```python
from build123d import *

# Parameters (mm, degrees)
F0_W      = 908.05
F0_H      = 34.925
F1_DEPTH  = 2032
F2_W      = 601.726
F2_H      = 615.442
F3_DEPTH  = 34.926
F8_DEPTH  = 926.592
F9_DEPTH  = 615.442
F11_DEPTH = 34.926
F13_DEPTH = 908.05
F15_DEPTH = 34.926
F17_W     = 506.7300000006
F17_H     = 34.925
F18_DEPTH = 831.596
F19_W     = 506.7300000008
F19_H     = 34.925
F20_DEPTH = 520.446


with BuildPart() as f1:
    # F0 (on Top) → F1 (new body)
    with BuildSketch(Plane.XY):
        with Locations((-454.025, 17.4625)):
            Rectangle(F0_W, F0_H)
    extrude(amount=F1_DEPTH)

    # F2 (on Front) → F3 (cut, through all)
    with BuildSketch(Plane.XZ):
        Polygon((-754.888, 1917.446), (-754.888, 990.854), (-153.162, 990.854), (-153.162, 1917.446), (-454.025, 1917.446), align=None)
        with Locations((-454.025, 510.921)):
            Rectangle(F2_W, F2_H)
    extrude(amount=-F3_DEPTH, mode=Mode.SUBTRACT)

    # F6 (on face) → F8 (join, through all)
    with BuildSketch(Plane(origin=(0, 0, 1917.446), x_dir=(1, 0, 0), z_dir=(0, 0, -1))):
        Polygon((-200.66, -17.4625), (-200.66, -34.925), (-186.8149014921, -24.003), (-176.911, -24.003), (-167.0070985079, -24.003), (-153.162, -34.925), (-153.162, -17.4625), (-153.162, 0), (-167.0070985079, -10.922), (-176.911, -10.922), (-186.8149014921, -10.922), (-200.66, 0), align=None)
        Polygon((-741.0429014921, -24.003), (-731.139, -24.003), (-721.2350985079, -24.003), (-707.39, -34.925), (-707.39, -17.4625), (-707.39, 0), (-721.2350985079, -10.922), (-731.139, -10.922), (-741.0429014921, -10.922), (-754.888, 0), (-754.888, -17.4625), (-754.888, -34.925), align=None)
    extrude(amount=F8_DEPTH)

    # F7 (on face) → F9 (join, through all)
    with BuildSketch(Plane.XY.offset(203.2)):
        Polygon((-200.66, 34.925), (-200.66, 17.4625), (-200.66, 0), (-186.8149014921, 10.922), (-176.911, 10.922), (-167.0070985079, 10.922), (-153.162, 0), (-153.162, 17.4625), (-153.162, 34.925), (-167.0070985079, 24.003), (-176.911, 24.003), (-186.8149014921, 24.003), align=None)
        Polygon((-721.2350985079, 24.003), (-731.139, 24.003), (-741.0429014921, 24.003), (-754.888, 34.925), (-754.888, 17.4625), (-754.888, 0), (-741.0429014921, 10.922), (-731.139, 10.922), (-721.2350985079, 10.922), (-707.39, 0), (-707.39, 17.4625), (-707.39, 34.925), align=None)
    extrude(amount=F9_DEPTH)

    # F10 (on Front) → F11 (cut, through all)
    with BuildSketch(Plane.XZ):
        Polygon((-754.888, 1917.446), (-454.025, 1616.583), (-153.162, 1917.446), (-200.66, 1917.446), (-707.39, 1917.446), align=None)
        Polygon((-153.162, 990.854), (-454.025, 1291.717), (-754.888, 990.854), (-200.66, 990.854), align=None)
        Polygon((-153.162, 818.642), (-200.66, 818.642), (-707.39, 818.642), (-754.888, 818.642), (-454.025, 517.779), align=None)
        Polygon((-754.888, 203.2), (-200.66, 203.2), (-153.162, 203.2), (-454.025, 504.063), align=None)
    extrude(amount=-F11_DEPTH, mode=Mode.SUBTRACT)


with BuildPart() as f13:
    # F12 (on Right) → F13 (new body, through all)
    with BuildSketch(Plane.YZ):
        Polygon((34.925, 1917.446), (0, 1917.446), (10.9219999999, 1903.6009014923), (10.922, 1883.7930985079), (0, 1869.948), (34.925, 1869.948), (24.003, 1883.793098508), (24.003, 1903.6009014921), align=None)
    extrude(amount=-F13_DEPTH)


with BuildPart() as f13b:
    # F12 (on Right) → F13, piece 2 (new body, through all)
    with BuildSketch(Plane.YZ):
        Polygon((10.922, 1004.6990985079), (0, 990.854), (34.925, 990.854), (24.0029999999, 1004.6990985081), (24.003, 1024.5069014921), (34.925, 1038.3520000001), (0, 1038.352), (10.922, 1024.5069014922), align=None)
    extrude(amount=-F13_DEPTH)


with BuildPart() as f13c:
    # F12 (on Right) → F13, piece 3 (new body, through all)
    with BuildSketch(Plane.YZ):
        Polygon((24.003, 784.9890985079), (24.003, 804.7969014922), (34.925, 818.642), (0, 818.642), (10.922, 804.796901492), (10.922, 784.9890985079), (1e-10, 771.1440000001), (34.925, 771.144), align=None)
    extrude(amount=-F13_DEPTH)


with BuildPart() as f13d:
    # F12 (on Right) → F13, piece 4 (new body, through all)
    with BuildSketch(Plane.YZ):
        Polygon((34.925, 203.2), (24.003, 217.0450985079), (24.003, 236.852901492), (34.925, 250.698), (0, 250.698), (10.922, 236.8529014921), (10.922, 217.0450985078), (0, 203.2), align=None)
    extrude(amount=-F13_DEPTH)


with BuildPart() as f15_tool:
    # F14 (on Front) → F15 (new body, through all)
    with BuildSketch(Plane.XZ):
        Polygon((-754.888, 818.642), (-754.888, 203.2), (-454.025, 504.063), (-153.162, 203.2), (-153.162, 818.642), (-454.025, 517.779), align=None)
        Polygon((-153.162, 1917.446), (-454.025, 1616.583), (-754.888, 1917.446), (-754.888, 990.854), (-454.025, 1291.717), (-153.162, 990.854), align=None)
    extrude(amount=-F15_DEPTH)


with BuildPart() as f13_1:
    add(f13.part)

    # F15: cut by f15_tool
    add(f15_tool.part, mode=Mode.SUBTRACT)


with BuildPart() as f13b_1:
    add(f13b.part)

    # F15: cut by f15_tool
    add(f15_tool.part, mode=Mode.SUBTRACT)


with BuildPart() as f13c_1:
    add(f13c.part)

    # F15: cut by f15_tool
    add(f15_tool.part, mode=Mode.SUBTRACT)


with BuildPart() as f13d_1:
    add(f13d.part)

    # F15: cut by f15_tool
    add(f15_tool.part, mode=Mode.SUBTRACT)


with BuildPart() as f1_1:
    add(f1.part)

    # F16: union F13, F13b, F13c, F13d
    add(f13_1.part)
    add(f13b_1.part)
    add(f13c_1.part)
    add(f13d_1.part)

    # F17 (on face) → F18 (join, through all)
    with BuildSketch(Plane.XY.offset(1038.352)):
        with Locations((-454.0250000003, 17.4625)):
            Rectangle(F17_W, F17_H)
    extrude(amount=F18_DEPTH)

    # F19 (on face) → F20 (join, through all)
    with BuildSketch(Plane.XY.offset(250.698)):
        with Locations((-454.0250000004, 17.4625)):
            Rectangle(F19_W, F19_H)
    extrude(amount=F20_DEPTH)


solid = f1_1.part
```
Geometry check sheet. Reference: the model listing, model coordinates, mm. A direction names the side the tool comes from. Coordinates: 2 decimals unless noted, no trailing zeros. Order: outer loops, then holes, each group sorted by start corner. A loop starts at its lowest first (then second) coordinate and runs counter-clockwise, first axis right, second up. Notation, with made-up numbers: (74.25, -29) - (133.25, -29) arc R18 ccw to (133.25, -6) - close; hole circle Ø2 at (47, 74.25). An arc over 180 degrees is marked (long way). Answer in a Markdown table with one row per item. Add a question column.
1. Access from +Z, -Z, +X, -X, +Y, -Y to the whole of each face (thin tool, end or side, straight path). Record for faces 1 (the face through (-729, 10.922, 534)), 2 (the face through (-763, 34.925, 776)).
2. Gauge pin test, flat end, axial feed: pin 1 Ø6 at (x, z) = (-406.5, 1893.5) entering from -Y. Record the tip position at first contact, or that the pin passes through.
3. Section check A-A (z = 1450.5). Enter the section's corners in (x, y) (3 decimals), plus the area to 3 significant figures.
4. Material ranges on L1, parallel to X at y = 26.5, z = 423; L2, parallel to X at y = 27.5, z = 577.5; L3, parallel to Z at x = -291, y = 6, recorded low to high. Write a range as [from, to].
5. Draft check along X on faces 3 (the face through (-176, 24.003, 510)), 4 (the face through (-460, 18, 0)), 5 (the face through (0, 17, 1030)). Enter one of: +X half, -X half, draft (parallel to the pull), parting line (faces both ways), or undercut.
Data:
| question | item | result |
|---|---|---|
| 1 | face 1 | -Y |
| 1 | face 2 | +Z, -Z, +X, -X, +Y |
| 2 | pin 1 | stops at y = 10.92 |
| 3 | outline | (-908.05, 0) - (-754.888, 0) - (-741.043, 10.922) - (-721.235, 10.922) - (-707.39, 0) - (-200.66, 0) - (-186.815, 10.922) - (-167.007, 10.922) - (-153.162, 0) - (0, 0) - (0, 34.925) - (-153.162, 34.925) - (-167.007, 24.003) - (-186.815, 24.003) - (-200.66, 34.925) - (-707.39, 34.925) - (-721.235, 24.003) - (-741.043, 24.003) - (-754.888, 34.925) - (-908.05, 34.925) - close |
| 3 | area | 30,200 mm² |
| 4 | L1 | x = [-908.05, -744.21], [-718.07, -189.98], [-163.84, 0] |
| 4 | L2 | x = [-908.05, -745.48], [-716.8, -191.25], [-162.57, 0] |
| 4 | L3 | z = [0, 210.81], [243.09, 778.75], [811.04, 998.46], [1030.75, 1877.55], [1909.84, 2032] |
| 5 | face 3 | undercut |
| 5 | face 4 | draft |
| 5 | face 5 | +X half |
